```python
from build123d import *

# Parameters (mm, degrees)
SKETCH11_R                                  = 2.5
QUADRADO_PF20_11_PERFIL_2020_V_SLOT_1_DEPTH = 200


with BuildPart() as part:
    # Sketch11 → Quadrado PF20-11 - PERFIL 2020 V-SLOT(1) (new body)
    with BuildSketch(Plane.YZ):
        with BuildLine():
            Line((-4.8, 10), (-3, 8.2))
            Line((-3, 8.2), (-5.5, 8.2))
            Line((-5.5, 8.2), (-5.5, 6.560660172))
            Line((-5.5, 6.560660172), (-2.939339828, 4))
            Line((-2.939339828, 4), (-0.3, 4))
            Line((-0.3, 4), (0, 3.7))
            Line((0, 3.7), (0.3, 4))
            Line((0.3, 4), (2.939339828, 4))
            Line((2.939339828, 4), (5.5, 6.560660172))
            Line((5.5, 6.560660172), (5.5, 8.2))
            Line((5.5, 8.2), (3, 8.2))
            Line((3, 8.2), (4.8, 10))
            Line((4.8, 10), (9, 10))
            ThreePointArc((9, 10), (9.707106781, 9.707106781), (10, 9))
            Line((10, 9), (10, 4.8))
            Line((10, 4.8), (8.2, 3))
            Line((8.2, 3), (8.2, 5.5))
            Line((8.2, 5.5), (6.560660172, 5.5))
            Line((6.560660172, 5.5), (4, 2.939339828))
            Line((4, 2.939339828), (4, 0.3))
            Line((4, 0.3), (3.7, 0))
            Line((3.7, 0), (4, -0.3))
            Line((4, -0.3), (4, -2.939339828))
            Line((4, -2.939339828), (6.560660172, -5.5))
            Line((6.560660172, -5.5), (8.2, -5.5))
            Line((8.2, -5.5), (8.2, -3))
            Line((8.2, -3), (10, -4.8))
            Line((10, -4.8), (10, -9))
            ThreePointArc((10, -9), (9.707106781, -9.707106781), (9, -10))
            Line((9, -10), (4.8, -10))
            Line((4.8, -10), (3, -8.2))
            Line((3, -8.2), (5.5, -8.2))
            Line((5.5, -8.2), (5.5, -6.560660172))
            Line((5.5, -6.560660172), (2.939339828, -4))
            Line((2.939339828, -4), (0.3, -4))
            Line((0.3, -4), (0, -3.7))
            Line((0, -3.7), (-0.3, -4))
            Line((-0.3, -4), (-2.939339828, -4))
            Line((-2.939339828, -4), (-5.5, -6.560660172))
            Line((-5.5, -6.560660172), (-5.5, -8.2))
            Line((-5.5, -8.2), (-3, -8.2))
            Line((-3, -8.2), (-4.8, -10))
            Line((-4.8, -10), (-9, -10))
            ThreePointArc((-9, -10), (-9.707106781, -9.707106781), (-10, -9))
            Line((-10, -9), (-10, -4.8))
            Line((-10, -4.8), (-8.2, -3))
            Line((-8.2, -3), (-8.2, -5.5))
            Line((-8.2, -5.5), (-6.560660172, -5.5))
            Line((-6.560660172, -5.5), (-4, -2.939339828))
            Line((-4, -2.939339828), (-4, -0.3))
            Line((-4, -0.3), (-3.7, 0))
            Line((-3.7, 0), (-4, 0.3))
            Line((-4, 0.3), (-4, 2.939339828))
            Line((-4, 2.939339828), (-6.560660172, 5.5))
            Line((-6.560660172, 5.5), (-8.2, 5.5))
            Line((-8.2, 5.5), (-8.2, 3))
            Line((-8.2, 3), (-10, 4.8))
            Line((-10, 4.8), (-10, 9))
            ThreePointArc((-10, 9), (-9.707106781, 9.707106781), (-9, 10))
            Line((-9, 10), (-4.8, 10))
        make_face()
        Circle(SKETCH11_R, mode=Mode.SUBTRACT)
    extrude(amount=QUADRADO_PF20_11_PERFIL_2020_V_SLOT_1_DEPTH)


solid = part.part
```
Geometry check sheet. Reference: the model listing, model coordinates, mm. Give positions to 0.01 mm unless a question says otherwise; leave off trailing zeros. Use CSV: the item, a comma, the result in double quotes. Start each with the question number.
Q1. Scan lines: probe 1 along Y at (x, z) = (43, -7.75); probe 2 along Z at (x, y) = (88, 0); probe 3 along Y at (x, z) = (190, 3.5). Record each from-to range of solid material in increasing order. Write a range as from..to.
Q2. Go/stop test with flat-tipped pins: pin 1 Ø3 at (x, z) = (125, -2.5) entering from -Y; pin 2 Ø4.5 at (y, z) = (0, 0) entering from +X (3 decimals); pin 3 Ø1 at (x, z) = (171.5, 3.5) entering from +Y; pin 4 Ø1.2 at (x, z) = (81.5, -4) entering from +Y. Record where each tip stops, or that it passes through.
Q3. Release check for a two-part mould opening along Y. For faces 1 (the face through (99, 7, 10)), 2 (the face through (99, -10, -7)), 3 (the face through (98.6, -0.54, -2.44)), 4 (the face through (99, 10, 7)) record: +Y half, -Y half, draft (parallel to the pull), parting line (faces both ways), or undercut.
Findings below:
1,probe 1,"y = -10..-5.5, 5.5..10"
1,probe 2,"z = -3.7..-2.5, 2.5..3.7"
1,probe 3,"y = -8.7..-8.2, -4.56..4.56, 8.2..8.7"
2,pin 1,"stops at y = -9.2"
2,pin 2,"passes through"
2,pin 3,"stops at y = 9.2"
2,pin 4,"stops at y = 9.8"
3,face 1,"draft"
3,face 2,"-Y half"
3,face 3,"undercut"
3,face 4,"+Y half"
